Autodesk Inventor part; units mm, degrees
ref_plane "YZ Plane" through (0, 0, 0) normal (1, 0, 0) x (0, 1, 0)
ref_plane "XZ Plane" through (0, 0, 0) normal (0, 1, 0) x (-1, 0, 0)
ref_plane "XY Plane" through (0, 0, 0) normal (0, 0, 1) x (1, 0, 0)
sketch "Sketch1" plane through (0, 0, 0) normal (0, 1, 0) x (-1, 0, 0)
  circle A0 centre (0, 0) radius 25
  dimension "d0" = 50
sketch "Sketch2" plane through (0, 0, 0) normal (0, 1, 0) x (-1, 0, 0)
  point P0 (0, 0)
extrude "Extrusion1" add sketch "Sketch1" along normal blind 10
sketch "Sketch3" plane through (0, 10, 0) normal (0, 1, 0) x (1, 0, 0)
  circle A0 centre (0, 0) radius 16
  dimension "d3" = 32
extrude "Extrusion2" cut sketch "Sketch3" against normal blind 5
sketch "Sketch4" plane through (0, 0, 0) normal (0, -1, 0) x (1, 0, 0)
  point P0 (0, 0)
sketch "Sketch5" plane through (0, 0, 0) normal (0, -1, 0) x (1, 0, 0)
  circle A0 centre (-17.7361, -11.5993) radius 2.5
  point P0 (0, 0)
  dimension "d6" = 5
extrude "Extrusion3" cut sketch "Sketch5" against normal blind 2
sketch "Sketch6" plane through (0, 0, 0) normal (0, -1, 0) x (1, 0, 0)
  circle A0 centre (-19.6243, -2.8324) radius 2.5
  point P0 (0, 0)
  dimension "d9" = 5
extrude "Extrusion4" cut sketch "Sketch6" against normal blind 2
sketch "Sketch7" plane through (0, 0, 0) normal (0, -1, 0) x (1, 0, 0)
  circle A0 centre (-8.6995, -18.343) radius 2.5
  point P0 (0, 0)
  dimension "d12" = 5
extrude "Extrusion5" cut sketch "Sketch7" against normal blind 2
sketch "Sketch8" plane through (0, 0, 0) normal (0, -1, 0) x (1, 0, 0)
  circle A0 centre (4.6532, -18.2082) radius 2.5
  point P0 (0, 0)
  dimension "d15" = 5
extrude "Extrusion6" cut sketch "Sketch8" against normal blind 2
sketch "Sketch9" plane through (0, 0, 0) normal (0, -1, 0) x (1, 0, 0)
  circle A0 centre (-5.3276, -8.7669) radius 2.5
  point P0 (0, 0)
  dimension "d18" = 5
extrude "Extrusion7" cut sketch "Sketch9" against normal blind 2
sketch "Sketch10" plane through (0, 0, 0) normal (0, -1, 0) x (1, 0, 0)
  circle A0 centre (9.6436, -10.2505) radius 2.5
  point P0 (0, 0)
  dimension "d21" = 5
extrude "Extrusion8" cut sketch "Sketch10" against normal blind 2
sketch "Sketch11" plane through (0, 0, 0) normal (0, -1, 0) x (1, 0, 0)
  circle A0 centre (-6.9461, 4.5858) radius 2.5
  point P0 (0, 0)
  dimension "d24" = 5
extrude "Extrusion9" cut sketch "Sketch11" against normal blind 2
sketch "Sketch12" plane through (0, 0, 0) normal (0, -1, 0) x (1, 0, 0)
  circle A0 centre (7.8902, 10.9249) radius 2.5
  point P0 (0, 0)
  dimension "d27" = 5
extrude "Extrusion10" cut sketch "Sketch12" against normal blind 2
sketch "Sketch13" plane through (0, 0, 0) normal (0, -1, 0) x (1, 0, 0)
  circle A0 centre (-13.4201, 11.5993) radius 2.5
  point P0 (0, 0)
  dimension "d30" = 5
extrude "Extrusion11" cut sketch "Sketch13" against normal blind 2
sketch "Sketch14" plane through (0, 0, 0) normal (0, -1, 0) x (1, 0, 0)
  circle A0 centre (17.871, 0) radius 2.5
  point P0 (0, 0)
  dimension "d33" = 5
extrude "Extrusion12" cut sketch "Sketch14" against normal blind 2
sketch "Sketch15" plane through (0, 0, 0) normal (0, -1, 0) x (1, 0, 0)
  circle A0 centre (0, 14.5665) radius 2.5
  point P0 (0, 0)
  dimension "d36" = 5
extrude "Extrusion13" cut sketch "Sketch15" against normal blind 2
properties part number "sprayer" material "PVC, Unplasticized"
Build history of the part. All positions in model axes, mm. A direction names the side the tool comes from. Coordinates: 2 decimals unless noted, no trailing zeros. Order: outer loops, then holes, each group sorted by start corner. A loop starts at its lowest first (then second) coordinate and runs counter-clockwise, first axis right, second up. Notation, with made-up numbers: (52, 46.25) - (105, 46.25) arc R14 cw to (105, 59.25) - close; hole circle Ø1 at (-32.5, 72). An arc over 180 degrees is marked (long way). Put each result on its own line as item: value.
1. Saw through at B-B (y = 9). Write the cut outline in (x, z).
Answer sheet:
outline: circle Ø50 at (0, 0); hole circle Ø32 at (0, 0)
2. Saw through at D-D (z = -4.5). Write the cut outline in (x, y).
Answer sheet:
outline: (-24.59, 0) - (-21.49, 0) - (-21.49, 2) - (-17.76, 2) - (-17.76, 0) - (24.59, 0) - (24.59, 10) - (15.35, 10) - (15.35, 5) - (-15.35, 5) - (-15.35, 10) - (-24.59, 10) - close
3. Pull direction Z, two halves, no side cores. Call faces 4 (the face through (0, 0, 0)), 5 (the face through (-23.846, 4.93, -7.509)), 6 (the face through (-18, 2, -12)): pulls with the +Z half, pulls with the -Z half, needs draft (parallel to the pull), parting line crosses it, or undercut.
Answer sheet:
face 4: needs draft
face 5: parting line crosses it
face 6: undercut
4. Tool access for faces 1 (the face through (-3.47, 7.54, 15.62)), 2 (the face through (0.3, 10, -16.3)), 3 (the face through (7.04, 0.99, -17.46)): list every direction of +Z, -Z, +X, -X, +Y, -Y with a clear straight run to the whole face (end or side of a thin tool).
Answer sheet:
face 1: +Y
face 2: +Z, -Z, +X, -X, +Y
face 3: -Y
5. Probe line 1 along X through (y, z) = (7.5, 0.5) (3 decimals); line 2 along Z through (x, y) = (-6, 1.25); line 3 along Y through (x, z) = (-4, 0). List the from-to ranges inside material, lowest first. Write a range as [from, to].
Answer sheet:
line 1: x = [-24.995, -15.992], [15.992, 24.995]
line 2: z = [-24.27, -11.17], [-6.36, 2.27], [6.9, 24.27]
line 3: y = [0, 5]
6. Saw through at C-C (y = 4). Write the cut outline in (x, z).
Answer sheet:
outline: circle Ø50 at (0, 0)
7. Saw through at A-A (x = 0). Write the cut outline in (y, z).
Answer sheet:
outline: (0, -25) - (10, -25) - (10, -16) - (5, -16) - (5, 16) - (10, 16) - (10, 25) - (0, 25) - (0, 17.07) - (2, 17.07) - (2, 12.07) - (0, 12.07) - close
8. Drop flat-ended pins along their axis: P1, Ø2, axis at y = 7, z = 3.5, coming from the +X side; P2, Ø6.5, axis at x = 0, z = 14.57, coming from the +Y side; P3, Ø16, axis at x = 3, z = -5.5, coming from the +Y side; P4, Ø1.5, axis at x = 19.5, y = 9, coming from the -Z side. Give the stop position or say it passes through.
Answer sheet:
P1: stops at x = 24.87
P2: stops at y = 10
P3: stops at y = 5
P4: stops at z = -16.54
